Geometry check sheet. Reference: the model listing, model coordinates, mm. Face numbers are marked on the shaded views. A direction names the side the tool comes from. Give positions to 0.01 mm unless a question says otherwise; leave off trailing zeros. Loops run counter-clockwise (first coordinate to the right, second up) from the corner with the lowest first, then second, coordinate; pieces in that order, holes last. Notation, with made-up numbers: (84, -25.5) -> (98, -25.5) arc R24 cw to (98, 3.5) -> close; hole circle Ø10 at (41.5, 3.25). An arc over 180 degrees is marked (long way). One line per item, written item: value. Start each with the question number.
(1) Sectioned sample at A-A, the plane x = 20. Record the cut outline in (y, z), then the cut area to 3 significant figures.
(2) Scan lines: line 1 along X through (y, z) = (2.3, 69.5); line 2 along X through (y, z) = (1, 7.5). Record each from-to range of solid material in increasing order. Write a range as from..to.
(3) Tool access check on the marked faces 1 and 2. Record the directions out of +Z, -Z, +X, -X, +Y, -Y that give a thin tool (end or side, any length) a straight path to the whole face; none if there is none.
(4) Sectioned sample at B-B, the plane z = 34.5. Record the cut outline in (x, y).
(5) Sectioned sample at D-D, the plane x = 64.5. Record the cut outline in (y, z).
(6) Gauge pin test, flat ends, axial feed: pin 1 Ø0.8 at (x, y) = (-4.5, 1) entering from +Z; pin 2 Ø8 at (x, z) = (48.5, 18.5) entering from +Y; pin 3 Ø10 at (x, z) = (13, 37.5) entering from -Y. Record the tip position at first contact, or that the pin passes through.
(7) Sectioned sample at C-C, the plane y = 0.5. Record the cut outline in (x, z), then the cut area to 3 significant figures.
Autodesk Inventor part; units mm, degrees
ref_plane "YZ Plane" through (0, 0, 0) normal (1, 0, 0) x (0, 1, 0)
ref_plane "XZ Plane" through (0, 0, 0) normal (0, 1, 0) x (-1, 0, 0)
ref_plane "XY Plane" through (0, 0, 0) normal (0, 0, 1) x (1, 0, 0)
sketch "Sketch1" plane through (0, 0, 0) normal (0, 1, 0) x (-1, 0, 0)
  line L0 (45.25, -45.25) -> (-45.25, -45.25)
  line L1 (-45.25, -45.25) -> (-45.25, 45.25)
  line L2 (-45.25, 45.25) -> (45.25, 45.25)
  line L3 (45.25, 45.25) -> (45.25, -45.25)
  line L4 (75.3, -75.3) -> (-75.3, -75.3)
  line L5 (-75.3, -75.3) -> (-75.3, 75.3)
  line L6 (-75.3, 75.3) -> (75.3, 75.3)
  line L7 (75.3, 75.3) -> (75.3, -75.3)
  line L8 (-77.3, 77.3) -> (-77.3, -77.3)
  line L9 (-77.3, -77.3) -> (77.3, -77.3)
  line L10 (77.3, -77.3) -> (77.3, 77.3)
  line L11 (77.3, 77.3) -> (-77.3, 77.3)
  point P0 (0, 0)
  point P1 (-45.25, 0)
  point P2 (0, -45.25)
  point P3 (-75.3, 0)
  point P4 (0, -75.3)
  dimension "d0" = 90.5
  dimension "d1" = 150.6
  dimension "d2" = 2
extrude "Extrusion1" add sketch "Sketch1" along normal blind 1.5 contours L4 L5 L6 L7
extrude "Extrusion2" add sketch "Sketch1" along normal blind 2.5 contours L11 L10 L9 L8
sketch "Sketch2" plane through (75.3, 1.5, 75.3) normal (0, 0, -1) x (-1, 0, 0)
  point P0 (75.3, -1.5)
sketch "Sketch3" plane through (-77.3, 0, 77.3) normal (0, 0, 1) x (1, 0, 0)
  line L0 (152.6, 2.5) -> (2, 2.5)
  line L1 (67.3, 2.5) -> (87.3, 2.5)
  line L2 (87.3, 2.5) -> (87.3, 0)
  line L3 (87.3, 0) -> (67.3, 0)
  line L4 (67.3, 0) -> (67.3, 2.5)
  line L5 (0, 0) -> (154.6, 0)
  line L6 (2, 1.5) -> (152.6, 1.5)
  line L7 (152.6, 1.5) -> (2, 1.5)
  line L8 (32.05, 1.5) -> (122.55, 1.5)
  line L9 (122.55, 1.5) -> (32.05, 1.5)
  point P0 (77.3, 0)
  point P1 (77.3, 0)
  point P2 (77.3, 0)
  dimension "d7" = 20
extrude "Extrusion3" cut sketch "Sketch3" against normal up to surface (2 mm away)
properties part number "15cmPasteMaskTemplate_3DPrint"
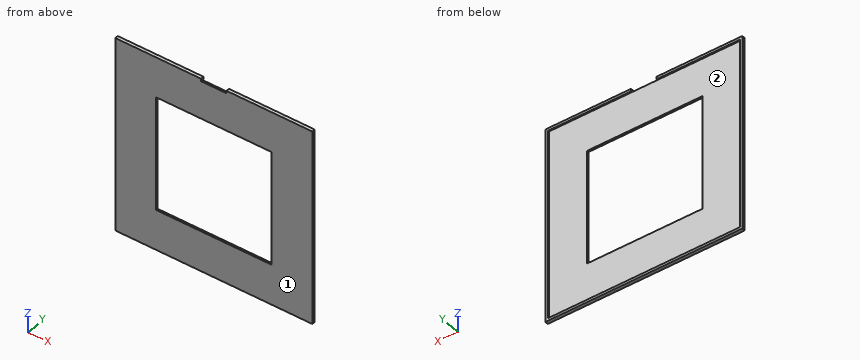
Calculated:
1. outline: (0, -77.3) -> (2.5, -77.3) -> (2.5, -75.3) -> (1.5, -75.3) -> (1.5, -45.25) -> (0, -45.25) -> close; (0, 45.25) -> (1.5, 45.25) -> (1.5, 75.3) -> (2.5, 75.3) -> (2.5, 77.3) -> (0, 77.3) -> close
1. area: 100 mm2
2. line 1: x = -77.3..-75.3, 75.3..77.3
2. line 2: x = -77.3..-45.25, 45.25..77.3
3. face 1: +Z, -Z, +X, -X, -Y
3. face 2: +Y
4. outline: (-77.3, 0) -> (-45.25, 0) -> (-45.25, 1.5) -> (-75.3, 1.5) -> (-75.3, 2.5) -> (-77.3, 2.5) -> close; (45.25, 0) -> (77.3, 0) -> (77.3, 2.5) -> (75.3, 2.5) -> (75.3, 1.5) -> (45.25, 1.5) -> close
5. outline: (0, -77.3) -> (2.5, -77.3) -> (2.5, -75.3) -> (1.5, -75.3) -> (1.5, 75.3) -> (2.5, 75.3) -> (2.5, 77.3) -> (0, 77.3) -> close
6. pin 1: stops at z = 75.3
6. pin 2: stops at y = 1.5
6. pin 3: passes through
7. outline: (-77.3, -77.3) -> (77.3, -77.3) -> (77.3, 77.3) -> (10, 77.3) -> (10, 75.3) -> (-10, 75.3) -> (-10, 77.3) -> (-77.3, 77.3) -> close; hole (-45.25, -45.25) -> (45.25, -45.25) -> (45.25, 45.25) -> (-45.25, 45.25) -> close
7. area: 15,700 mm2
